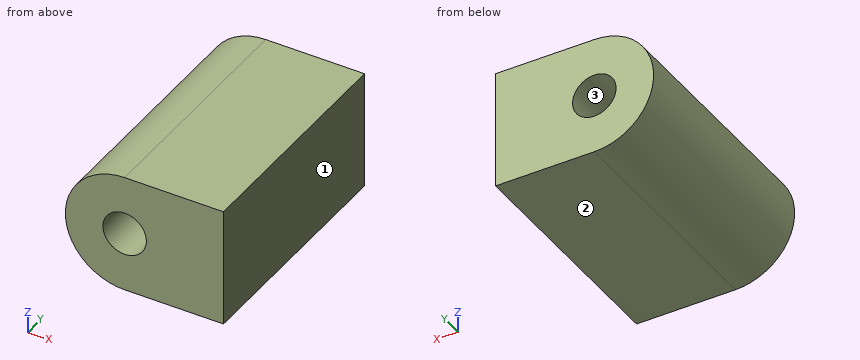
from build123d import *

# Parameters (mm, degrees)
SKETCH1_R           = 2.75
BOSS_EXTRUDE1_DEPTH = 30


with BuildPart() as part:
    # Sketch1 → Boss-Extrude1 (new body)
    with BuildSketch(Plane(origin=(0, 0, 0), x_dir=(1, 0, 0), z_dir=(0, 1, 0))):
        with BuildLine():
            Line((0, 7.5), (-12.5, 7.5))
            ThreePointArc((-12.5, 7.5), (-20, 0), (-12.5, -7.5))
            Line((-12.5, -7.5), (0, -7.5))
            Line((0, -7.5), (0, 7.5))
        make_face()
        with Locations(Location((-12.5, 0, 0), (0, 0, 270))):
            Circle(SKETCH1_R, mode=Mode.SUBTRACT)
    extrude(amount=BOSS_EXTRUDE1_DEPTH)


solid = part.part
Can you work these out from the model? Positions are in its coordinate system, mm. Face numbers are marked on the shaded views. Round coordinates to 2 decimals unless told otherwise and drop trailing zeros. Order: outer loops, then holes, each group sorted by start corner. A loop starts at its lowest first (then second) coordinate and runs counter-clockwise, first axis right, second up. Notation, with made-up numbers: (62.25, 53.25) - (75.25, 53.25) arc R21 ccw to (75.25, 73.25) - close; hole circle Ø11 at (87.25, -9.75). An arc over 180 degrees is marked (long way). Answer in a Markdown table with one row per item.
(1) For P1, Ø1, axis at y = 6, z = 4.5, coming from the -X side, with a flat end and sliding along its axis, tell me the tip position at first contact or that it passes through.
From the geometry:
| item | result |
|---|---|
| P1 | stops at x = -18.84 |
(2) Please list where these lines run through material, in increasing order: L1, parallel to X at y = 7.5, z = 0; L2, parallel to Z at x = -11.5, y = 23.5; L3, parallel to X at y = 12.75, z = -2.5. Write a range as from..to.
From the geometry:
| item | result |
|---|---|
| L1 | x = -20..-15.25, -9.75..0 |
| L2 | z = -7.5..-2.56, 2.56..7.5 |
| L3 | x = -19.57..-13.65, -11.35..0 |
(3) Suppose I cut it at A-A, the plane z = 0. Please give me the cut outline in (x, y), plus the area to 3 significant figures.
From the geometry:
| item | result |
|---|---|
| outline | (-20, 0) - (-15.25, 0) - (-15.25, 30) - (-20, 30) - close; (-9.75, 0) - (0, 0) - (0, 30) - (-9.75, 30) - close |
| area | 435 mm2 |
(4) If we mould it in two halves opening along Z, with no side actions, what happens to the marked faces 1, 2 and 3? For each: released by +Z, released by -Z, zero draft, split by the parting line, or undercut.
From the geometry:
| item | result |
|---|---|
| face 1 | zero draft |
| face 2 | released by -Z |
| face 3 | undercut |
(5) Suppose I cut it at D-D, the plane z = -4.5. Please give me the cut outline in (x, y), plus the area to 3 significant figures.
From the geometry:
| item | result |
|---|---|
| outline | (-18.5, 0) - (0, 0) - (0, 30) - (-18.5, 30) - close |
| area | 555 mm2 |
(6) Suppose I cut it at B-B, the plane y = 10. Please give me the cut outline in (x, z), plus the area to 3 significant figures.
From the geometry:
| item | result |
|---|---|
| outline | (-12.5, -7.5) - (0, -7.5) - (0, 7.5) - (-12.5, 7.5) arc R7.5 ccw to start; hole circle Ø5.5 at (-12.5, 0) |
| area | 252 mm2 |
(7) Suppose I cut it at C-C, the plane z = 2.25. Please give me the cut outline in (x, y).
From the geometry:
| item | result |
|---|---|
| outline | (-19.65, 0) - (-14.08, 0) - (-14.08, 30) - (-19.65, 30) - close; (-10.92, 0) - (0, 0) - (0, 30) - (-10.92, 30) - close |
